CAD build for the part. Positions are in the model's coordinates, mm. A direction names the side the tool comes from. Give positions to 0.01 mm unless a question says otherwise; leave off trailing zeros. Loops run counter-clockwise (first coordinate to the right, second up) from the corner with the lowest first, then second, coordinate; pieces in that order, holes last.
Item 1: Mould opens along X. For faces 3 (the cylindrical face through (-11.09, 0.783, -52.276)), 4 (the cylindrical face through (-37.41, 0.78, -11.41)), 5 (the flat face through (-25.4, 1, -27)) say: released by +X, released by -X, zero draft, split by the parting line, or undercut.
Item 2: Saw through at D-D on x = -7.5. Give the cut face in (y, z).
Item 3: Saw through at C-C on z = -1. Give the cut face in (x, y), plus the area to 3 significant figures.
Item 4: Probe probe 1 along Z at (x, y) = (-31.75, 0.7); probe 2 along Z at (x, y) = (-7.5, 0.45). List the from-to ranges inside material, lowest first.
Item 5: Saw through at B-B on x = -31.75. Give the cut face in (y, z), plus the area to 3 significant figures.
Item 6: Saw through at A-A on y = 0.6. Give the number of separate pieces and of enclosed holes in the cut face, plus the area to 3 significant figures.
Item 7: Which spindle directions (+Z, -Z, +X, -X, +Y, -Y) get a long thin tool onto all of the face, cutting with end or side? Do faces 1 (the flat face through (-5, 1, -6.35)), 2 (the cylindrical face through (-33.749, 0.783, -14.917)). Say none if no direction does.
Item 8: Drop a flat-ended pin along its axis: P1, Ø0.8, axis at y = 0.5, z = -27, coming from the +X side. Give the stop position or say it passes through.
Autodesk Inventor part; units mm, degrees
ref_plane "YZ Plane" through (0, 0, 0) normal (1, 0, 0) x (0, 1, 0)
ref_plane "XZ Plane" through (0, 0, 0) normal (0, 1, 0) x (-1, 0, 0)
ref_plane "XY Plane" through (0, 0, 0) normal (0, 0, 1) x (1, 0, 0)
sketch "gusset" plane through (0, 0, 0) normal (0, 0, 1) x (1, 0, 0)
  circle A0 centre (-8.9225, 14.8571) radius 2.1844
  circle A1 centre (-21.6225, 14.8571) radius 2.1844
  arc A2 (-21.6225, 21.2071) -> (-21.6225, 8.5071) centre (-21.6225, 14.8571) ccw
  arc A3 (-5.1125, 19.9371) -> (-8.9225, 21.2071) centre (-8.9225, 14.8571) ccw
  line L0 (16.4775, 0.5696) -> (16.4775, -20.0679)
  line L1 (3.7775, -20.1515) -> (3.7775, -4.1929)
  line L2 (2.5075, -1.6529) -> (-10.1925, 7.8721)
  line L3 (-21.6225, 8.5071) -> (-12.0975, 8.5071)
  line L4 (-21.6225, 21.2071) -> (-8.9225, 21.2071)
  arc A4 (16.4775, 0.5696) -> (13.9375, 5.6496) centre (10.1275, 0.5696) ccw
  line L5 (-5.1125, 19.9371) -> (13.9375, 5.6496)
  circle A5 centre (-21.6232, -35.9429) radius 2.1844
  circle A6 centre (-8.9225, -35.9429) radius 2.1844
  line L6 (-21.6246, -29.5943) -> (-8.9205, -29.5916)
  line L7 (-21.6233, -42.2916) -> (-7.3358, -42.2916)
  arc A7 (-21.6246, -29.5943) -> (-21.6233, -42.2916) centre (-21.6232, -35.9429) ccw
  circle A8 centre (10.1275, 0.5696) radius 2.0955
  circle A9 centre (10.1275, -20.0679) radius 2.0955
  arc A10 (3.7775, -4.1929) -> (2.5075, -1.6529) centre (0.6025, -4.1929) ccw
  arc A11 (-10.1925, 7.8721) -> (-12.0975, 8.5071) centre (-12.0975, 5.3321) ccw
  arc A12 (-7.3358, -42.2916) -> (16.4487, -20.6722) centre (-7.3358, -18.3986) ccw
  arc A13 (16.4487, -20.6722) -> (16.4775, -20.0679) centre (10.1275, -20.0679) ccw
  arc A14 (-8.9205, -29.5916) -> (3.7028, -20.8361) centre (-7.3358, -18.3986) ccw
  arc A15 (3.7028, -20.8361) -> (3.7775, -20.1515) centre (0.6025, -20.1515) ccw
  point P0 (-7.0147, -10.522)
  point P1 (16.4775, -20.3474)
  point P2 (3.7775, -20.4691)
  point P3 (4.4125, 12.7933)
  dimension "d0" = 12.7
  dimension "d2" = 12.7
  dimension "d3" = 4.191
  dimension "d4" = 3.175
  dimension "d8" = 12.7
  dimension "d12" = 14.2875
  dimension "d13" = 6.35
  dimension "d14" = 15.875
  dimension "d15" = 3.175
sketch "Sketch1" plane through (0, 0, 0) normal (0, 1, 0) x (-1, 0, 0)
  circle A0 centre (12.7, 0) radius 2.1844
  circle A1 centre (0, 0) radius 2.1844
  arc A2 (0, 6.35) -> (0, -6.35) centre (0, 0) ccw
  arc A3 (16.51, 5.08) -> (12.7, 6.35) centre (12.7, 0) ccw
  line L0 (38.1, -14.2875) -> (38.1, -34.925)
  line L1 (25.4, -35.0086) -> (25.4, -19.05)
  line L2 (24.13, -16.51) -> (11.43, -6.985)
  line L3 (0, -6.35) -> (9.525, -6.35)
  line L4 (0, 6.35) -> (12.7, 6.35)
  arc A4 (38.1, -14.2875) -> (35.56, -9.2075) centre (31.75, -14.2875) ccw
  line L5 (16.51, 5.08) -> (35.56, -9.2075)
  circle A5 centre (-0.0007, -50.8) radius 2.1844
  circle A6 centre (12.7, -50.8) radius 2.1844
  line L6 (-0.0021, -44.4514) -> (12.702, -44.4486)
  line L7 (-0.0008, -57.1486) -> (14.2867, -57.1486)
  arc A7 (-0.0021, -44.4514) -> (-0.0008, -57.1486) centre (-0.0007, -50.8) ccw
  circle A8 centre (31.75, -14.2875) radius 2.0955
  circle A9 centre (31.75, -34.925) radius 2.0955
  arc A10 (25.4, -19.05) -> (24.13, -16.51) centre (22.225, -19.05) ccw
  arc A11 (11.43, -6.985) -> (9.525, -6.35) centre (9.525, -9.525) ccw
  arc A12 (14.2867, -57.1486) -> (38.0712, -35.5292) centre (14.2867, -33.2557) ccw
  arc A13 (38.0712, -35.5292) -> (38.1, -34.925) centre (31.75, -34.925) ccw
  arc A14 (12.702, -44.4486) -> (25.3253, -35.6931) centre (14.2867, -33.2557) ccw
  arc A15 (25.3253, -35.6931) -> (25.4, -35.0086) centre (22.225, -35.0086) ccw
extrude "Extrusion1" add sketch "Sketch1" along normal blind 1.5875
properties part number "Rear Gusset" material "Acetal Resin, White"
Results below:
1. face 3: undercut
1. face 4: released by -X
1. face 5: released by +X
2. outline: (0, -57.15) - (1.59, -57.15) - (1.59, -44.45) - (0, -44.45) - close; (0, -6.35) - (1.59, -6.35) - (1.59, 6.35) - (0, 6.35) - close
3. outline: (-24.62, 0) - (-14.64, 0) - (-14.64, 1.59) - (-24.62, 1.59) - close; (-10.76, 0) - (-1.94, 0) - (-1.94, 1.59) - (-10.76, 1.59) - close; (1.94, 0) - (6.27, 0) - (6.27, 1.59) - (1.94, 1.59) - close
3. area: 36.7 mm2
4. probe 1: z = -49.56 to -37.02, -32.83 to -16.38, -12.19 to -6.35
4. probe 2: z = -57.15 to -44.45, -6.35 to 6.35
5. outline: (0, -49.56) - (1.59, -49.56) - (1.59, -37.02) - (0, -37.02) - close; (0, -32.83) - (1.59, -32.83) - (1.59, -16.38) - (0, -16.38) - close; (0, -12.19) - (1.59, -12.19) - (1.59, -6.35) - (0, -6.35) - close
5. area: 55.3 mm2
6. separate pieces: 1
6. enclosed holes: 6
6. area: 1,270 mm2
7. face 1: +X, +Y, -Y
7. face 2: +Y, -Y
8. P1: stops at x = -25.4
